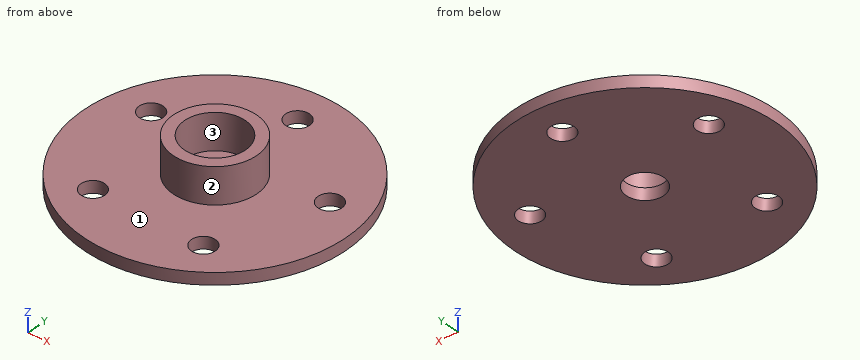
from build123d import *

# Parameters (mm, degrees)
SKETCH_1_R      = 22
SKETCH_1_R_2    = 3.15
SKETCH_1_R_3    = 2
EXTRUDE_1_DEPTH = 2
SKETCH_2_R      = 7
SKETCH_2_R_2    = 5.1
EXTRUDE_3_DEPTH = 6


with BuildPart() as part:
    # 草图1 → 凸台-拉伸1 (new body)
    with BuildSketch(Plane.XY):
        Circle(SKETCH_1_R)
        Circle(SKETCH_1_R_2, mode=Mode.SUBTRACT)
        with Locations((0, 16)):
            Circle(SKETCH_1_R_3, mode=Mode.SUBTRACT)
        with Locations((15.216904261, 4.94427191)):
            Circle(SKETCH_1_R_3, mode=Mode.SUBTRACT)
        with Locations((9.404564037, -12.94427191)):
            Circle(SKETCH_1_R_3, mode=Mode.SUBTRACT)
        with Locations((-9.404564037, -12.94427191)):
            Circle(SKETCH_1_R_3, mode=Mode.SUBTRACT)
        with Locations((-15.216904261, 4.94427191)):
            Circle(SKETCH_1_R_3, mode=Mode.SUBTRACT)
    extrude(amount=EXTRUDE_1_DEPTH)

    # 草图2 → 凸台-拉伸3 (add)
    with BuildSketch(Plane.XY.offset(2)):
        Circle(SKETCH_2_R)
        Circle(SKETCH_2_R_2, mode=Mode.SUBTRACT)
    extrude(amount=EXTRUDE_3_DEPTH)


solid = part.part
Source: CAD feature listing. Evaluate the final solid. Frame: model axes, mm. Face numbers are marked on the shaded views. Coordinates: 2 decimals unless noted, no trailing zeros. Loops run counter-clockwise (first coordinate to the right, second up) from the corner with the lowest first, then second, coordinate; pieces in that order, holes last. Notation, with made-up numbers: (25.25, 31.25) - (68.25, 31.25) arc R20 ccw to (68.25, 40.25) - close; hole circle Ø9 at (79.5, -24). An arc over 180 degrees is marked (long way). One line per item, written item: value. Start each with the question number.
1. Section A-A (y = 0). Return the cut outline in (x, z).
2. Mould query, pull axis X, two halves, no side actions, for the marked faces 1, 2 and 3. Classes: pulls with the +X half, pulls with the -X half, needs draft (parallel to the pull), parting line crosses it, or undercut.
3. Contact query for flat-ended pins moving along their axis: P1, Ø5.5, axis at x = 0, y = 0, coming from the +Z side; P2, Ø5, axis at x = 15.22, y = 4.94, coming from the +Z side; P3, Ø2, axis at x = 4, z = 5.5, coming from the -Y side; P4, Ø1.5, axis at y = -10, z = 2.5, coming from the +X side. Output: stop coordinate, or through.
4. Section D-D (z = 6.75). Return the cut outline in (x, y), and give its area (3 significant figures).
5. Ray query, L1, parallel to Y at x = 0, z = 0.55; L2, parallel to Y at x = 0, z = 6.55; L3, parallel to X at y = -3, z = 4.5. Return the intervals inside material, ascending.
6. Section B-B (x = 0). Return the cut outline in (y, z).
7. Section C-C (y = -12). Return the cut outline in (x, z).
Verdict:
1. outline: (-22, 0) - (-3.15, 0) - (-3.15, 2) - (-5.1, 2) - (-5.1, 8) - (-7, 8) - (-7, 2) - (-22, 2) - close; (3.15, 0) - (22, 0) - (22, 2) - (7, 2) - (7, 8) - (5.1, 8) - (5.1, 2) - (3.15, 2) - close
2. face 1: needs draft
2. face 2: parting line crosses it
2. face 3: undercut
3. P1: passes through
3. P2: stops at z = 2
3. P3: stops at y = -6.32
3. P4: stops at x = 19.87
4. outline: circle Ø14 at (0, 0); hole circle Ø10.2 at (0, 0)
4. area: 72.2 mm2
5. L1: y = -22 to -3.15, 3.15 to 14, 18 to 22
5. L2: y = -7 to -5.1, 5.1 to 7
5. L3: x = -6.32 to -4.12, 4.12 to 6.32
6. outline: (-22, 0) - (-3.15, 0) - (-3.15, 2) - (-5.1, 2) - (-5.1, 8) - (-7, 8) - (-7, 2) - (-22, 2) - close; (3.15, 0) - (14, 0) - (14, 2) - (7, 2) - (7, 8) - (5.1, 8) - (5.1, 2) - (3.15, 2) - close; (18, 0) - (22, 0) - (22, 2) - (18, 2) - close
7. outline: (-18.44, 0) - (-11.17, 0) - (-11.17, 2) - (-18.44, 2) - close; (-7.64, 0) - (7.64, 0) - (7.64, 2) - (-7.64, 2) - close; (11.17, 0) - (18.44, 0) - (18.44, 2) - (11.17, 2) - close
